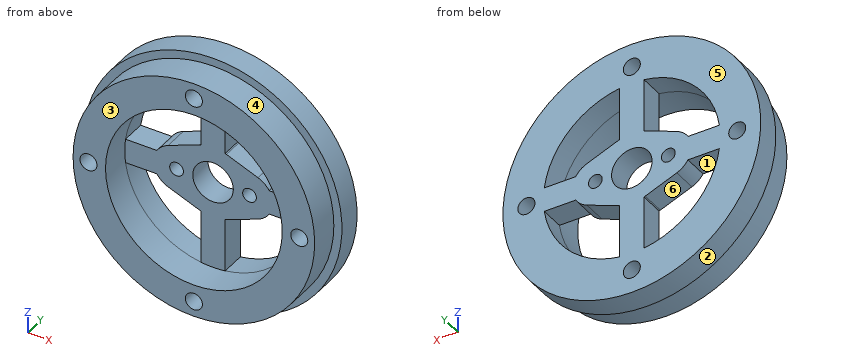
from build123d import *

# Parameters (mm, degrees)
HOLE_WIZARD_1_7_1_7_1_D     = 1.7
HOLE_WIZARD_1_7_1_7_1_DEPTH = 6
HOLE_WIZARD_2_1_2_1_1_D     = 2.1
CUT_EXTRUDE_START           = -10
CUT_EXTRUDE_1_DEPTH         = 10


with BuildPart() as part:
    # 草图2 → 旋转1 (revolve)
    with BuildSketch(Plane.XY, mode=Mode.PRIVATE) as revolve_1_sk:
        Polygon((2.5, 6.8), (15.9, 6.8), (15.9, 3.8), (14.9, 3.8), (14.9, 0), (10.9, 0), (10.9, 3.8), (2.5, 3.8), align=None)
    revolve(revolve_1_sk.sketch.rotate(Axis((0, 0, 0), (0, 1, 0)), 90), axis=Axis((0, 0, 0), (0, 1, 0)))

    # Ø1.7 (1.7) 直径孔1
    with Locations(Plane(origin=(0, 6.8, 0), x_dir=(1, 0, 0), z_dir=(0, 1, 0))):
        with Locations((-4.5, 0), (4.5, 0)):
            Hole(HOLE_WIZARD_1_7_1_7_1_D / 2, depth=HOLE_WIZARD_1_7_1_7_1_DEPTH)

    # Ø2.1 (2.1) 直径孔1 (through all)
    with Locations(Plane(origin=(0, 0, 0), x_dir=(-1, 0, 0), z_dir=(0, -1, 0))):
        with Locations((-13, 0), (0, 13), (13, 0), (0, -13)):
            Hole(HOLE_WIZARD_2_1_2_1_1_D / 2)

    # 草图9 → 切除-拉伸1 (cut)
    with BuildSketch(Plane.XZ.offset(-3.8).offset(CUT_EXTRUDE_START)):
        with BuildLine():
            Line((-5.545, 2.65150429), (-1.65, 4.186585721))
            ThreePointArc((-1.65, 4.186585721), (-1.575249358, 4.215280472), (-1.5, 4.242640687))
            Line((-1.5, 4.242640687), (-1.5, 10.796295661))
            ThreePointArc((-1.5, 10.796295661), (-7.707463915, 7.707463915), (-10.796295661, 1.5))
            Line((-10.796295661, 1.5), (-6.923324163, 1.5))
            ThreePointArc((-6.923324163, 1.5), (-6.327240722, 2.187165138), (-5.545, 2.65150429))
        make_face()
        with BuildLine():
            ThreePointArc((-5.545, -2.65150429), (-6.327240722, -2.187165138), (-6.923324163, -1.5))
            Line((-6.923324163, -1.5), (-10.796295661, -1.5))
            ThreePointArc((-10.796295661, -1.5), (-7.707463915, -7.707463915), (-1.5, -10.796295661))
            Line((-1.5, -10.796295661), (-1.5, -4.242640687))
            ThreePointArc((-1.5, -4.242640687), (-1.575249358, -4.215280472), (-1.65, -4.186585721))
            Line((-1.65, -4.186585721), (-5.545, -2.65150429))
        make_face()
        with BuildLine():
            Line((1.5, 10.796295661), (1.5, 4.242640687))
            ThreePointArc((1.5, 4.242640687), (1.575249358, 4.215280472), (1.65, 4.186585721))
            Line((1.65, 4.186585721), (5.545, 2.65150429))
            ThreePointArc((5.545, 2.65150429), (6.327240722, 2.187165138), (6.923324163, 1.5))
            Line((6.923324163, 1.5), (10.796295661, 1.5))
            ThreePointArc((10.796295661, 1.5), (7.707463915, 7.707463915), (1.5, 10.796295661))
        make_face()
        with BuildLine():
            ThreePointArc((1.65, -4.186585721), (1.575249358, -4.215280472), (1.5, -4.242640687))
            Line((1.5, -4.242640687), (1.5, -10.796295661))
            ThreePointArc((1.5, -10.796295661), (7.707463915, -7.707463915), (10.796295661, -1.5))
            Line((10.796295661, -1.5), (6.923324163, -1.5))
            ThreePointArc((6.923324163, -1.5), (6.327240722, -2.187165138), (5.545, -2.65150429))
            Line((5.545, -2.65150429), (1.65, -4.186585721))
        make_face()
    extrude(amount=CUT_EXTRUDE_1_DEPTH, mode=Mode.SUBTRACT)


solid = part.part
The model under review builds one solid part; all positions refer to its coordinate system, in mm. Face numbers are marked on the shaded views. A direction names the side the tool comes from. Coordinates: 2 decimals unless noted, no trailing zeros. Loops run counter-clockwise (first coordinate to the right, second up) from the corner with the lowest first, then second, coordinate; pieces in that order, holes last. Notation, with made-up numbers: (49, 76) -> (58, 76) arc R31 ccw to (58, 101) -> close; hole circle Ø2 at (38, -9.5). An arc over 180 degrees is marked (long way). Use a Markdown table: item, result. Add a question column.
1. Add section C-C on y = 3.25. Write out the cut boundary in (x, z).
2. Add section D-D on z = -8.5. Write out the cut boundary in (x, y), plus the area to 3 significant figures.
3. To check wall thickness, follow line 1 (Z direction, x = -5.5, y = 4.75); line 2 (Y direction, x = -13.5, z = 7); line 3 (Z direction, x = 7, y = 6). State the ranges of each line that lie inside material, in increasing order.
4. Clearance check with flat-ended pins moving along their axes: pin 1 Ø2 at (y, z) = (3, -4.5) entering from +X; pin 2 Ø2 at (x, y) = (-6, 3.5) entering from +Z; pin 3 Ø3.5 at (y, z) = (6, -6) entering from +X. State where each tip first meets the part, or that it passes through.
5. Machinability: for the marked faces 4, 5 and 6, which of the approach directions +Z, -Z, +X, -X, +Y, -Y give a long, thin tool a straight path to every point of the face, cutting with its end or side? Answer none if there is none.
6. Draft analysis for pull direction Z (two halves, no side actions). For the marked faces 1, 2 and 3, state which applies: pulls with the +Z half, pulls with the -Z half, needs draft (parallel to the pull), parting line crosses it, or undercut.
7. Add section A-A on z = 0. Give the number of separate pieces and of enclosed holes in the cut face, plus the area to 3 significant figures.
Returned:
| question | item | result |
|---|---|---|
| 1 | outline | circle Ø29.8 at (0, 0); hole circle Ø2.1 at (-13, 0); hole circle Ø21.8 at (0, 0); hole circle Ø2.1 at (0, -13); hole circle Ø2.1 at (0, 13); hole circle Ø2.1 at (13, 0) |
| 2 | outline | (-13.44, 3.8) -> (-12.24, 3.8) -> (-12.24, 0) -> (-6.82, 0) -> (-6.82, 6.8) -> (-13.44, 6.8) -> close; (-1.5, 3.8) -> (1.5, 3.8) -> (1.5, 6.8) -> (-1.5, 6.8) -> close; (6.82, 0) -> (12.24, 0) -> (12.24, 3.8) -> (13.44, 3.8) -> (13.44, 6.8) -> (6.82, 6.8) -> close |
| 2 | area | 89.8 mm² |
| 3 | line 1 | z = -14.92 to -9.41, -2.67 to 2.67, 9.41 to 14.92 |
| 3 | line 2 | y = 3.8 to 6.8 |
| 3 | line 3 | z = -14.28 to -8.36, -1.5 to 1.5, 8.36 to 14.28 |
| 4 | pin 1 | stops at x = 15.41 |
| 4 | pin 2 | stops at z = 15.08 |
| 4 | pin 3 | stops at x = 15.32 |
| 5 | face 4 | -Y |
| 5 | face 5 | +Z, -Z, +X, -X, +Y |
| 5 | face 6 | +Y, -Y |
| 6 | face 1 | undercut |
| 6 | face 2 | parting line crosses it |
| 6 | face 3 | needs draft |
| 7 | separate pieces | 6 |
| 7 | enclosed holes | 0 |
| 7 | area | 72.0 mm² |
